Design review of the part built by this model. Coordinates are the model's own, in mm. Face numbers are marked on the shaded views. Give positions to 0.01 mm unless a question says otherwise; leave off trailing zeros. Write each loop counter-clockwise with the first axis right and the second up, starting at its lowest first coordinate (ties: lowest second). Pieces come first, ordered by that corner, then holes. Notation, with made-up numbers: M 48,53.5 L 60,53.5 A16 cw 60,78.5 Z; hole C -3.75,5 d6. An arc over 180 degrees is marked long. Answer in a Markdown table with one row per item.
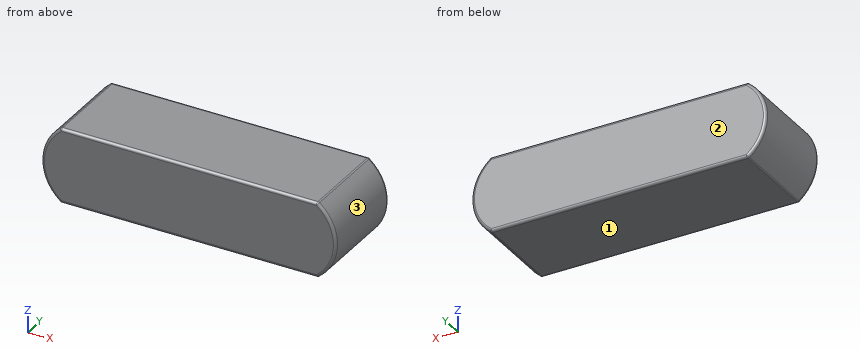
```python
from build123d import *

# Parameters (mm, degrees)
F1_DEPTH = 34
F2_R     = 1


with BuildPart() as f1:
    # F0 (on Front) → F1 (new body)
    with BuildSketch(Plane.XZ):
        with BuildLine():
            Line((-48, -14), (48, -14))
            ThreePointArc((48, -14), (55.003177, 0), (48, 14))
            Line((48, 14), (-48, 14))
            ThreePointArc((-48, 14), (-55.003177, 0), (-48, -14))
        make_face()
    extrude(amount=F1_DEPTH)

    # F2
    f2_edges = [f1.edges().sort_by_distance(p)[0] for p in [
        (-55.003177, -34, 0),
        (0, -34, -14),
        (55.003177, -34, 0),
        (0, -34, 14),
        (-55.003177, 0, 0),
        (0, 0, -14),
        (55.003177, 0, 0),
        (0, 0, 14),
        (48, -17, 14),
        (-48, -17, 14),
        (-48, -17, -14),
        (48, -17, -14),
    ]]
    fillet(f2_edges, radius=F2_R)


solid = f1.part
```
1) To check wall thickness, follow probe 1 along X at (y, z) = (-4.5, 0.5); probe 2 along X at (y, z) = (-22.5, -3.5); probe 3 along Z at (x, y) = (48.5, -8.5). State the ranges of each line that lie inside material, in increasing order. Write a range as [from, to].
Geometry says:
| item | result |
|---|---|
| probe 1 | [-55, 55] |
| probe 2 | [-54.65, 54.65] |
| probe 3 | [-13.61, 13.61] |
2) Add section A-A (y = -30.5). Write out the cut boundary in (x, z), and give its area (3 significant figures).
Geometry says:
| item | result |
|---|---|
| outline | M -48.28,-13.79 A1 ccw -47.66,-14 L 47.66,-14 A1 ccw 48.28,-13.79 A17.5 ccw 48.28,13.79 A1 ccw 47.66,14 L -47.66,14 A1 ccw -48.28,13.79 A17.5 ccw Z |
| area | 2,960 mm^2 |
3) Insertion check: P1, Ø12, axis at y = -16, z = 11, coming from the -X side. The pin has a flat end and moves straight along its axis. Give the tip position at first contact, or say it passes through.
Geometry says:
| item | result |
|---|---|
| P1 | x = -54.27 |
4) The part is to be moulded in two halves that separate along Z. For the marked faces 1, 2 and 3, say which applies: released by +Z, released by -Z, zero draft, split by the parting line, or undercut.
Geometry says:
| item | result |
|---|---|
| face 1 | released by -Z |
| face 2 | zero draft |
| face 3 | split by the parting line |
